```python
from build123d import *

# Parameters (mm, degrees)
F0_W     = 9.398
F0_H     = 9.398
F1_DEPTH = 19.05
F2_R     = 38.1
F3_DEPTH = 7.62


with BuildPart() as f1:
    # F0 (on Front) → F1 (new body)
    with BuildSketch(Plane.XZ):
        Rectangle(F0_W, F0_H)
    extrude(amount=F1_DEPTH)

    # F2 (on face) → F3 (join)
    with BuildSketch(Plane.XZ.offset(19.05)):
        Circle(F2_R)
        with BuildLine():
            Line((-31.400349, -4.699), (-4.699, -4.699))
            Line((-4.699, -4.699), (-4.699, -31.400349))
            ThreePointArc((-4.699, -31.400349), (-22.45064, -22.45064), (-31.400349, -4.699))
        make_face(mode=Mode.SUBTRACT)
        with BuildLine():
            Line((4.699, -31.400349), (4.699, -4.699))
            Line((4.699, -4.699), (31.400349, -4.699))
            ThreePointArc((31.400349, -4.699), (22.45064, -22.45064), (4.699, -31.400349))
        make_face(mode=Mode.SUBTRACT)
        with BuildLine():
            ThreePointArc((-31.400349, 4.699), (-22.45064, 22.45064), (-4.699, 31.400349))
            Line((-4.699, 31.400349), (-4.699, 4.699))
            Line((-4.699, 4.699), (-31.400349, 4.699))
        make_face(mode=Mode.SUBTRACT)
        with BuildLine():
            Line((31.400349, 4.699), (4.699, 4.699))
            Line((4.699, 4.699), (4.699, 31.400349))
            ThreePointArc((4.699, 31.400349), (22.45064, 22.45064), (31.400349, 4.699))
        make_face(mode=Mode.SUBTRACT)
    extrude(amount=F3_DEPTH)


solid = f1.part
```
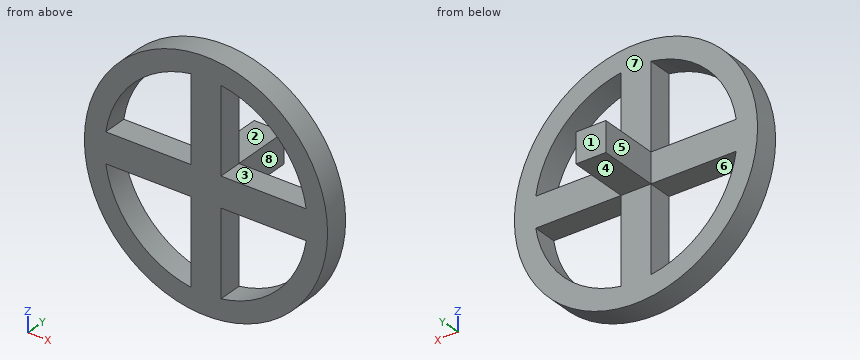
The model under review builds one solid part; all positions refer to its coordinate system, in mm. Face numbers are marked on the shaded views. A direction names the side the tool comes from. Give positions to 0.01 mm unless a question says otherwise; leave off trailing zeros. Write each loop counter-clockwise with the first axis right and the second up, starting at its lowest first coordinate (ties: lowest second). Pieces come first, ordered by that corner, then holes. Notation, with made-up numbers: M 7,32 L 18,32 A35 cw 18,70 Z; hole C 54.5,83.5 d8. An arc over 180 degrees is marked long. Answer in a Markdown table with one row per item.
Item 1: Tool access review of the marked faces 1, 2, 3, 4 and 5: name each direction out of +Z, -Z, +X, -X, +Y, -Y from which nothing blocks a thin tool from reaching the whole face with its end or side.
Check sheet entries:
| item | result |
|---|---|
| face 1 | +Z, -Z, +X, -X, +Y |
| face 2 | +Z, +X, -X, +Y |
| face 3 | +Y, -Y |
| face 4 | -Z, +X, -X, +Y |
| face 5 | +Z, -Z, -X, +Y |
Item 2: Add section A-A on z = 0. Give the boundary of the cut face in (x, y), plus the area to 3 significant figures.
Check sheet entries:
| item | result |
|---|---|
| outline | M -38.1,-26.67 L 38.1,-26.67 L 38.1,-19.05 L 4.7,-19.05 L 4.7,0 L -4.7,0 L -4.7,-19.05 L -38.1,-19.05 Z |
| area | 760 mm2 |
Item 3: For line 1 along Z through (x, y) = (28, -22.5); line 2 along X through (y, z) = (-24, 5); line 3 along X through (y, z) = (-20, -15), list the stretches that pass through material, from the lowest coordinate up.
Check sheet entries:
| item | result |
|---|---|
| line 1 | -25.84 to -14.97, -4.7 to 4.7, 14.97 to 25.84 |
| line 2 | -37.77 to -31.35, -4.7 to 4.7, 31.35 to 37.77 |
| line 3 | -35.02 to -27.98, -4.7 to 4.7, 27.98 to 35.02 |
Item 4: Draft analysis for pull direction X (two halves, no side actions). For the marked faces 6, 7 and 8, state which applies: +X half, -X half, draft (parallel to the pull), parting line (faces both ways), or undercut.
Check sheet entries:
| item | result |
|---|---|
| face 6 | undercut |
| face 7 | draft |
| face 8 | +X half |
Item 5: Add section D-D on x = 21. Give the boundary of the cut face in (y, z).
Check sheet entries:
| item | result |
|---|---|
| outline | M -26.67,-31.79 L -19.05,-31.79 L -19.05,-23.81 L -26.67,-23.81 Z; M -26.67,-4.7 L -19.05,-4.7 L -19.05,4.7 L -26.67,4.7 Z; M -26.67,23.81 L -19.05,23.81 L -19.05,31.79 L -26.67,31.79 Z |
Item 6: Add section B-B on x = 0. Give the boundary of the cut face in (y, z).
Check sheet entries:
| item | result |
|---|---|
| outline | M -26.67,-38.1 L -19.05,-38.1 L -19.05,-4.7 L 0,-4.7 L 0,4.7 L -19.05,4.7 L -19.05,38.1 L -26.67,38.1 Z |
Item 7: For P1, Ø6, axis at x = -25, z = -15.5, coming from the +Y side; P2, Ø2.5, axis at x = 12.5, y = -22, coming from the -Z side; P3, Ø6, axis at y = -20.5, z = 16.5, coming from the +X side, all flat-tipped, find the tip position at first contact; note any pin that passes through.
Check sheet entries:
| item | result |
|---|---|
| P1 | y = -19.05 |
| P2 | z = -36.4 |
| P3 | x = 35.63 |
Item 8: Add section C-C on z = 13.5. Give the boundary of the cut face in (x, y), plus the area to 3 significant figures.
Check sheet entries:
| item | result |
|---|---|
| outline | M -35.63,-26.67 L -28.74,-26.67 L -28.74,-19.05 L -35.63,-19.05 Z; M -4.7,-26.67 L 4.7,-26.67 L 4.7,-19.05 L -4.7,-19.05 Z; M 28.74,-26.67 L 35.63,-26.67 L 35.63,-19.05 L 28.74,-19.05 Z |
| area | 177 mm2 |
